Here's how the part is built. I have some questions about the finished solid (model axes, mm). A direction names the side the tool comes from. Give positions to 0.01 mm unless a question says otherwise; leave off trailing zeros. Loops run counter-clockwise (first coordinate to the right, second up) from the corner with the lowest first, then second, coordinate; pieces in that order, holes last.
Q1. If we section it at B-B (z = -9.5): Please give me the cut outline in (x, y).
Q2. I need wall thicknesses on line 1 (Y direction, x = 0, z = -4); line 2 (X direction, y = -2.9, z = -4.25); line 3 (Y direction, x = 19.5, z = -2.75). Which ranges of each line are inside material? Lowest first, please.
Q3. If we section it at A-A (z = -4.25): Please give me the cut outline in (x, y), plus the area to 3 significant figures.
Q4. If we section it at D-D (x = -17): Please give me the cut outline in (y, z), plus the area to 3 significant figures.
Q5. If we section it at C-C (x = -8.5): Please give me the cut outline in (y, z).
Q6. For faces 4 (the face through (0, 0, -12)), 5 (the face through (-18.28, -2.63, -3.8)), which set-ups out of +Z, -Z, +X, -X, +Y, -Y let a thin tool reach every point of the face, with its end or its side?
Q7. Will these pins go through, and if not, where does the flat tip stop? P1, Ø3, axis at x = -6, y = 2.5, coming from the -Z side; P2, Ø4, axis at y = -1, z = -6, coming from the +X side; P3, Ø4, axis at x = -19.5, y = -2.9, coming from the +Z side; P4, Ø1.5, axis at x = 19.5, y = -2.9, coming from the +Z side.
Q8. We'd pull the mould along X, two halves only. Please class faces 1 (the face through (24.28, -0.08, -5.72)), 2 (the face through (0, 4, 0)), 3 (the face through (20.72, -2.63, -3.8)): +X half, -X half, draft (parallel to the pull), parting line (faces both ways), or undercut.
from build123d import *

# Parameters (mm, degrees)
SKETCH_1_R                = 5.4
EXTRUDE_1_DEPTH           = 45
EXTRUDE_3_DEPTH           = 5.4
M8X1_0_TAPPED_HOLE1_D     = 7
M8X1_0_TAPPED_HOLE1_DEPTH = 13
M8X1_0_TAPPED_HOLE1_TIP   = 2.103012167
M3_TAPPED_HOLE1_D         = 2.5
M3_TAPPED_HOLE1_DEPTH     = 7.5
M3_TAPPED_HOLE1_TIP       = 0.751075774
CHAMFER_2_SIZE            = 0.5
SKETCH_9_R                = 4.25
CUT_EXTRUDE_5_DEPTH       = 2
CHAMFER_3_SIZE            = 0.5
SKETCH_10_R               = 6.935438506
CUT_EXTRUDE_1_DEPTH       = 86
HOLE_WIZARD_M8_1_D        = 6.8
HOLE_WIZARD_M8_1_DEPTH    = 9
HOLE_WIZARD_M8_1_TIP      = 2.042926105
FILLET_1_R                = 2


with BuildPart() as part:
    # 草图1 → 拉伸1 (new body)
    with BuildSketch(Plane.XY):
        with Locations(Location((0, 0, 0), (0, 0, 180))):
            Circle(SKETCH_1_R)
    extrude(amount=EXTRUDE_1_DEPTH)

    # 草图4 → 拉伸3 (add, symmetric)
    with BuildSketch(Plane.XZ):
        with BuildLine():
            Line((-22, 0), (22, 0))
            Line((22, 0), (28, -15.05119142))
            ThreePointArc((28, -15.05119142), (0, -12), (-28, -15.05119142))
            Line((-28, -15.05119142), (-22, 0))
        make_face()
    extrude(amount=EXTRUDE_3_DEPTH, both=True)

    # M8x1.0 Tapped Hole1
    with Locations(Plane.XY.offset(45)):
        with Locations((0, 0)):
            Hole(M8X1_0_TAPPED_HOLE1_D / 2, depth=M8X1_0_TAPPED_HOLE1_DEPTH)
            with Locations((0, 0, -(M8X1_0_TAPPED_HOLE1_DEPTH + M8X1_0_TAPPED_HOLE1_TIP / 2))):  # 118° drill point
                Cone(0, M8X1_0_TAPPED_HOLE1_D / 2, M8X1_0_TAPPED_HOLE1_TIP, mode=Mode.SUBTRACT)

    # M3 Tapped Hole1
    with Locations(Plane(origin=(-19.5, -2.9, 0), x_dir=(0, 1, 0), z_dir=(0, 0, 1))):
        with Locations((0, 0), (0, -39)):
            Hole(M3_TAPPED_HOLE1_D / 2, depth=M3_TAPPED_HOLE1_DEPTH)
            with Locations((0, 0, -(M3_TAPPED_HOLE1_DEPTH + M3_TAPPED_HOLE1_TIP / 2))):  # 118° drill point
                Cone(0, M3_TAPPED_HOLE1_D / 2, M3_TAPPED_HOLE1_TIP, mode=Mode.SUBTRACT)

    # 倒角2
    chamfer_2_edges = [part.edges().sort_by_distance(p)[0] for p in [
        (5.4, 0, 45),
    ]]
    chamfer(chamfer_2_edges, length=CHAMFER_2_SIZE)

    # 草图9 → 拉伸5 (cut)
    with BuildSketch(Plane.XY.offset(45)):
        Circle(SKETCH_9_R)
    extrude(amount=-CUT_EXTRUDE_5_DEPTH, mode=Mode.SUBTRACT)

    # 倒角3
    chamfer_3_edges = [part.edges().sort_by_distance(p)[0] for p in [
        (-4.25, 0, 45),
        (3.5, 0, 43),
    ]]
    chamfer(chamfer_3_edges, length=CHAMFER_3_SIZE)

    # 草图10 → 切除-拉伸1 (cut)
    with BuildSketch(Plane.XY):
        Circle(SKETCH_10_R)
    extrude(amount=CUT_EXTRUDE_1_DEPTH, mode=Mode.SUBTRACT)

    # M8 螺纹孔1
    with Locations(Plane.XY):
        with Locations((0, 0)):
            Hole(HOLE_WIZARD_M8_1_D / 2, depth=HOLE_WIZARD_M8_1_DEPTH)
            with Locations((0, 0, -(HOLE_WIZARD_M8_1_DEPTH + HOLE_WIZARD_M8_1_TIP / 2))):  # 118° drill point
                Cone(0, HOLE_WIZARD_M8_1_D / 2, HOLE_WIZARD_M8_1_TIP, mode=Mode.SUBTRACT)

    # 圆角1
    fillet_1_edges = [part.edges().sort_by_distance(p)[0] for p in [
        (-28, 0, -15.05119142),
        (28, 0, -15.05119142),
    ]]
    fillet(fillet_1_edges, radius=FILLET_1_R)


solid = part.part
Check sheet entries:
1. outline: (-25.79, -5.4) - (25.79, -5.4) - (25.79, 5.4) - (-25.79, 5.4) - close; hole circle Ø5.14 at (0, 0)
2. line 1: y = -5.4 to -3.4, 3.4 to 5.4
2. line 2: x = -23.69 to -20.75, -18.25 to -1.77, 1.77 to 18.25, 20.75 to 23.69
2. line 3: y = -5.4 to -4.15, -1.65 to 5.4
3. outline: (-23.69, -5.4) - (23.69, -5.4) - (23.69, 5.4) - (-23.69, 5.4) - close; hole circle Ø2.5 at (-19.5, -2.9); hole circle Ø6.8 at (0, 0); hole circle Ø2.5 at (19.5, -2.9)
3. area: 466 mm2
4. outline: (-5.4, -13.12) - (5.4, -13.12) - (5.4, 0) - (-5.4, 0) - close
4. area: 142 mm2
5. outline: (-5.4, -12.28) - (5.4, -12.28) - (5.4, 0) - (-5.4, 0) - close
6. face 4: -Z, +Y, -Y
6. face 5: +Z
7. P1: stops at z = -12.22
7. P2: stops at x = 25.19
7. P3: stops at z = 0
7. P4: stops at z = -7.8
8. face 1: +X half
8. face 2: draft
8. face 3: undercut
